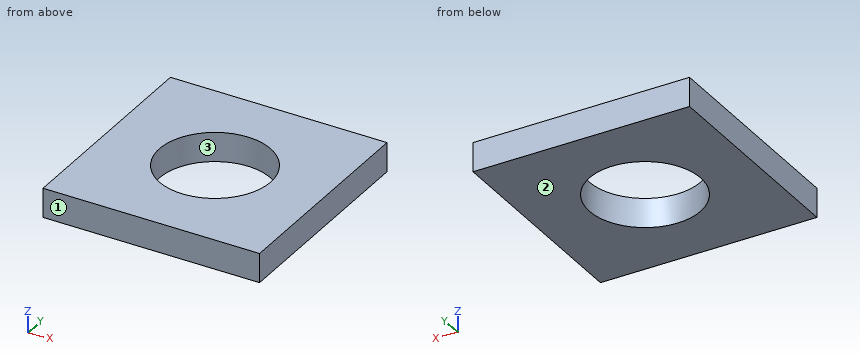
from build123d import *

# Parameters (mm, degrees)
F0_W     = 37
F0_H     = 37
F0_R     = 9.5
F1_DEPTH = 5
F2_ANGLE = 90


with BuildPart() as f1:
    # F0 (on Front) → F1 (new body)
    with BuildSketch(Plane.XZ):
        Rectangle(F0_W, F0_H)
        Circle(F0_R, mode=Mode.SUBTRACT)
    extrude(amount=F1_DEPTH)


with BuildPart() as f1_1:
    # F2: moved
    add(f1.part.rotate(Axis((0, 0, 18.5), (-1, 0, 0)), F2_ANGLE))


with BuildPart() as f1_2:
    # F3: moved
    add(f1_1.part.moved(Location((16, 32, -21))))


solid = f1_2.part
Model file for the job. Use its own axes, mm. Face numbers are marked on the shaded views. Give positions to 0.01 mm unless a question says otherwise; leave off trailing zeros. Order: outer loops, then holes, each group sorted by start corner. A loop starts at its lowest first (then second) coordinate and runs counter-clockwise, first axis right, second up. Notation, with made-up numbers: (25, 77.5) -> (42, 77.5) arc R32 ccw to (42, 108.5) -> close; hole circle Ø7 at (50, 11). An arc over 180 degrees is marked (long way). Use CSV: the item, a comma, the result in double quotes.
1. Mould opens along Y. For the marked faces 1, 2 and 3 say: +Y half, -Y half, draft (parallel to the pull), parting line (faces both ways), or undercut.
Outcome:
face 1,"-Y half"
face 2,"draft"
face 3,"undercut"
2. Band-saw the part on A-A, the plane y = 13.5. Give the cut face in (x, z).
Outcome:
outline,"(-2.5, -2.5) -> (6.5, -2.5) -> (6.5, 2.5) -> (-2.5, 2.5) -> close; (25.5, -2.5) -> (34.5, -2.5) -> (34.5, 2.5) -> (25.5, 2.5) -> close"
3. Band-saw the part on C-C, the plane z = 1.9. Give the cut face in (x, y).
Outcome:
outline,"(-2.5, -5) -> (34.5, -5) -> (34.5, 32) -> (-2.5, 32) -> close; hole circle Ø19 at (16, 13.5)"
4. Band-saw the part on B-B, the plane x = 16. Give the cut face in (y, z).
Outcome:
outline,"(-5, -2.5) -> (4, -2.5) -> (4, 2.5) -> (-5, 2.5) -> close; (23, -2.5) -> (32, -2.5) -> (32, 2.5) -> (23, 2.5) -> close"
5. Drill centre lines: line 1 along Y through (x, z) = (16, -0.1); line 2 along X through (y, z) = (13, -1.1); line 3 along Y through (x, z) = (9.5, -1.8). Where is each one in solid material? Low to high. Write a range as from..to.
Outcome:
line 1,"-5..4, 23..32"
line 2,"-2.5..6.51, 25.49..34.5"
line 3,"-5..6.57, 20.43..32"
